Read the model definition and answer for the solid it produces. Units are mm, in the model's axes. Face numbers are marked on the shaded views. A direction names the side the tool comes from. Round coordinates to 2 decimals unless told otherwise and drop trailing zeros. Order: outer loops, then holes, each group sorted by start corner. A loop starts at its lowest first (then second) coordinate and runs counter-clockwise, first axis right, second up. Notation, with made-up numbers: (-38, 69) -> (11, 69) arc R23 cw to (11, 92) -> close; hole circle Ø10 at (35.25, 4). An arc over 180 degrees is marked (long way). Use a Markdown table: item, result. Add a question column.
1. Section D-D, the plane x = 18 is taken. Give the vertices of the cut face in (y, z), then the cut area to 3 significant figures.
2. Given pin 1 (5 mm diameter, centred on y = -8, z = 14.5, fed in from -X); pin 2 (1.6 mm diameter, centred on x = 15.68, y = 15.52, fed in from +Z); pin 3 (12 mm diameter, centred on x = 4.5, y = 9, fed in from +Z); pin 4 (6.5 mm diameter, centred on x = -28.5, y = 15, fed in from -Z), each flat-ended and moving along its own axis, determine where each tip first touches the part or whether it passes through.
3. The mould has two halves that part along Y. Classify the marked faces 1, 2, 3 and 4: +Y half, -Y half, draft (parallel to the pull), parting line (faces both ways), or undercut.
4. For the marked faces 5, 6, 7 and 8, determine the directions among +Z, -Z, +X, -X, +Y, -Y from which every point of the face is accessible in a straight line to the end or side of a thin tool.
5. Section A-A, the plane z = 23.25 is taken. Give the vertices of the cut face in (x, y).
6. Section B-B, the plane x = 28.5 is taken. Give the vertices of the cut face in (y, z), then the cut area to 3 significant figures.
7. Consider L1, parallel to Y at x = -28.5, z = 20; L2, parallel to X at y = 6, z = 7.75. Determine where each line is inside the solid, lowest interval first. Write a range as [from, to].
8. Section C-C, the plane z = 11 is taken. Give the vertices of the cut face in (x, y).
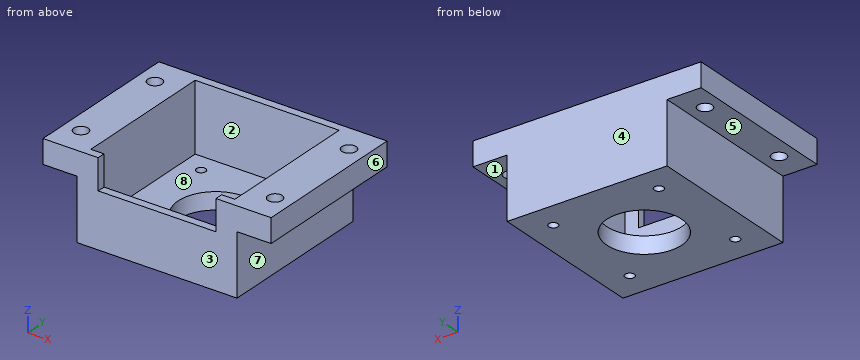
```python
from build123d import *

# Parameters (mm, degrees)
SKETCH_1_W               = 47
SKETCH_1_H               = 47
EXTRUDE_1_DEPTH          = 53
SKETCH_2_W               = 42.3
SKETCH_2_H               = 42.3
CUT_EXTRUDE_1_DEPTH      = 48
CUT_EXTRUDE_2_DEPTH      = 59.38236035
CUT_EXTRUDE_2_DEPTH_BACK = 59.38236035
SKETCH_3_R               = 11
SKETCH_3_R_2             = 1.35
SKETCH_7_W               = 28
SKETCH_7_H               = 47.225094233
CUT_EXTRUDE_5_DEPTH      = 47.5
SKETCH_20_W              = 10
SKETCH_20_H              = 47
SKETCH_20_R              = 2.1
EXTRUDE_2_DEPTH          = 7
SKETCH_23_W              = 34.56360228
SKETCH_23_H              = 9
CUT_EXTRUDE_8_DEPTH      = 2.35


with BuildPart() as part:
    # Эскиз1 → Бобышка-Вытянуть1 (new body)
    with BuildSketch(Plane.XY):
        Rectangle(SKETCH_1_W, SKETCH_1_H)
    extrude(amount=EXTRUDE_1_DEPTH)

    # Эскиз2 → Вырез-Вытянуть1 (cut)
    with BuildSketch(Plane.XY.offset(53)):
        Rectangle(SKETCH_2_W, SKETCH_2_H)
    extrude(amount=-CUT_EXTRUDE_1_DEPTH, mode=Mode.SUBTRACT)

    # Эскиз3 → Вырез-Вытянуть2 (cut, two sides: drawn at the far end of the back side and taken through both)
    with BuildSketch(Plane.XY.offset(5).offset(-CUT_EXTRUDE_2_DEPTH_BACK)):
        with Locations((0.178742266, 0.022649375)):
            Circle(SKETCH_3_R)
        with Locations((-15.321257734, 15.522649375)):
            Circle(SKETCH_3_R_2)
        with Locations(Location((15.678742266, 15.522649375, 0), (0, 0, 180))):
            Circle(SKETCH_3_R_2)
        with Locations((15.678742266, -15.477350625)):
            Circle(SKETCH_3_R_2)
        with Locations(Location((-15.321257734, -15.477350625, 0), (0, 0, 180))):
            Circle(SKETCH_3_R_2)
    extrude(amount=CUT_EXTRUDE_2_DEPTH + CUT_EXTRUDE_2_DEPTH_BACK, mode=Mode.SUBTRACT)

    # Эскиз7 → Вырез-Вытянуть5 (cut)
    with BuildSketch(Plane(origin=(23.5, 0, 0), x_dir=(0, 0, -1), z_dir=(1, 0, 0))):
        with Locations((-39, -0.112547117)):
            Rectangle(SKETCH_7_W, SKETCH_7_H)
    extrude(amount=-CUT_EXTRUDE_5_DEPTH, mode=Mode.SUBTRACT)

    # Эскиз20 → Бобышка-Вытянуть2 (add)
    # profile 1 of 2: a face of its own
    with BuildSketch(Plane.XY.offset(25)):
        with Locations((-28.5, 0)):
            Rectangle(SKETCH_20_W, SKETCH_20_H)
        with Locations((-28.5, 15)):
            Circle(SKETCH_20_R, mode=Mode.SUBTRACT)
        with Locations(Location((-28.5, -15, 0), (0, 0, 180))):
            Circle(SKETCH_20_R, mode=Mode.SUBTRACT)
    # profile 2 of 2: a face of its own
    with BuildSketch(Plane.XY.offset(25)):
        with Locations((28.5, 0)):
            Rectangle(SKETCH_20_W, SKETCH_20_H)
        with Locations((28.5, -15)):
            Circle(SKETCH_20_R, mode=Mode.SUBTRACT)
        with Locations(Location((28.5, 15, 0), (0, 0, 180))):
            Circle(SKETCH_20_R, mode=Mode.SUBTRACT)
    extrude(amount=-EXTRUDE_2_DEPTH)

    # Эскиз23 → Вырез-Вытянуть8 (cut)
    with BuildSketch(Plane(origin=(0, -23.5, 0), x_dir=(-1, 0, 0), z_dir=(0, -1, 0))):
        with Locations((0, -20.5)):
            Rectangle(SKETCH_23_W, SKETCH_23_H)
    extrude(amount=-CUT_EXTRUDE_8_DEPTH, mode=Mode.SUBTRACT)


solid = part.part
```
Verdict:
| question | item | result |
|---|---|---|
| 1 | outline | (-23.5, 0) -> (23.5, 0) -> (23.5, 25) -> (21.15, 25) -> (21.15, 5) -> (-21.15, 5) -> (-21.15, 25) -> (-23.5, 25) -> close |
| 1 | area | 329 mm2 |
| 2 | pin 1 | stops at x = -23.5 |
| 2 | pin 2 | passes through |
| 2 | pin 3 | stops at z = 5 |
| 2 | pin 4 | stops at z = 18 |
| 3 | face 1 | draft |
| 3 | face 2 | undercut |
| 3 | face 3 | -Y half |
| 3 | face 4 | +Y half |
| 4 | face 5 | -Z, -X, +Y, -Y |
| 4 | face 6 | +Z, -Z, +X, +Y, -Y |
| 4 | face 7 | -Z, +X, +Y, -Y |
| 4 | face 8 | +Z |
| 5 | outline | (-33.5, -23.5) -> (-17.28, -23.5) -> (-17.28, -21.15) -> (-21.15, -21.15) -> (-21.15, 21.15) -> (21.15, 21.15) -> (21.15, -21.15) -> (17.28, -21.15) -> (17.28, -23.5) -> (33.5, -23.5) -> (33.5, 23.5) -> (-33.5, 23.5) -> close; hole circle Ø4.2 at (-28.5, -15); hole circle Ø4.2 at (-28.5, 15); hole circle Ø4.2 at (28.5, -15); hole circle Ø4.2 at (28.5, 15) |
| 6 | outline | (-23.5, 18) -> (-17.1, 18) -> (-17.1, 25) -> (-23.5, 25) -> close; (-12.9, 18) -> (12.9, 18) -> (12.9, 25) -> (-12.9, 25) -> close; (17.1, 18) -> (23.5, 18) -> (23.5, 25) -> (17.1, 25) -> close |
| 6 | area | 270 mm2 |
| 7 | L1 | y = [-23.5, -17.1], [-12.9, 12.9], [17.1, 23.5] |
| 7 | L2 | x = [-23.5, -21.15], [21.15, 23.5] |
| 8 | outline | (-23.5, -23.5) -> (23.5, -23.5) -> (23.5, 23.5) -> (-23.5, 23.5) -> close; hole (-21.15, -21.15) -> (21.15, -21.15) -> (21.15, 21.15) -> (-21.15, 21.15) -> close |
